from build123d import *

# Parameters (mm, degrees)
EXTRUDE_1_DEPTH     = 10
FILLET_1_R          = 5
CUT_EXTRUDE_1_DEPTH = 58.341084747
CUT_EXTRUDE_2_DEPTH = 59.557663888


with BuildPart() as part:
    # 草图1 → 凸台-拉伸1 (new body)
    with BuildSketch(Plane(origin=(0, 0, 0), x_dir=(0, 0, -1), z_dir=(1, 0, 0))):
        Polygon((0, 0), (52, 0), (52, 25), (49, 25), (49, 3), (3, 3), (3, 25), (0, 25), align=None)
    extrude(amount=EXTRUDE_1_DEPTH)

    # 圆角1
    fillet_1_edges = [part.edges().sort_by_distance(p)[0] for p in [
        (5, 3, -3),
        (5, 3, -49),
        (5, 0, -52),
        (5, 0, 0),
    ]]
    fillet(fillet_1_edges, radius=FILLET_1_R)

    # 草图2 → 切除-拉伸1 (cut, through all)
    with BuildSketch(Plane(origin=(0, 3, 0), x_dir=(1, 0, 0), z_dir=(0, 1, 0))):
        with BuildLine():
            Line((7.5, 33.5), (7.5, 18.5))
            ThreePointArc((7.5, 18.5), (5, 16), (2.5, 18.5))
            Line((2.5, 18.5), (2.5, 33.5))
            ThreePointArc((2.5, 33.5), (5, 36), (7.5, 33.5))
        make_face()
    extrude(amount=-CUT_EXTRUDE_1_DEPTH, mode=Mode.SUBTRACT)

    # 草图3 → 切除-拉伸2 (cut, through all)
    with BuildSketch(Plane.XY):
        with BuildLine():
            Line((7.5, 17.5), (7.5, 12.5))
            ThreePointArc((7.5, 12.5), (5, 10), (2.5, 12.5))
            Line((2.5, 12.5), (2.5, 17.5))
            ThreePointArc((2.5, 17.5), (5, 20), (7.5, 17.5))
        make_face()
    extrude(amount=-CUT_EXTRUDE_2_DEPTH, mode=Mode.SUBTRACT)


solid = part.part
Work out the finished part from the listing and answer in its coordinate system (mm). A direction names the side the tool comes from. Coordinates: 2 decimals unless noted, no trailing zeros. Loops run counter-clockwise (first coordinate to the right, second up) from the corner with the lowest first, then second, coordinate; pieces in that order, holes last. Notation, with made-up numbers: (21.25, -12) -> (80.25, -12) arc R10 cw to (80.25, 5) -> close; hole circle Ø8 at (-31, 86.5). An arc over 180 degrees is marked (long way). Answer as CSV lines item,"result".
1) For faces 4 (the face through (4.9, 20.2, -3)), 5 (the face through (2.5, 15, -50)), 6 (the face through (5, 2, -16)), determine the directions among +Z, -Z, +X, -X, +Y, -Y from which every point of the face is accessible in a straight line to the end or side of a thin tool.
A:
face 4,"+X, -X, +Y"
face 5,"+Z, -Z"
face 6,"+Y, -Y"
2) The part is cut by section A-A (x = 6.5). Give the vertices of the cut face in (y, z), and give its area (3 significant figures).
A:
outline,"(0, -47) arc R5 ccw to (5, -52) -> (10.5, -52) -> (10.5, -49) -> (8, -49) arc R5 cw to (3, -44) -> (3, -35.5) -> (0, -35.5) -> close; (0, -16.5) -> (3, -16.5) -> (3, -8) arc R5 cw to (8, -3) -> (10.5, -3) -> (10.5, 0) -> (5, 0) arc R5 ccw to (0, -5) -> close; (19.5, -52) -> (25, -52) -> (25, -49) -> (19.5, -49) -> close; (19.5, -3) -> (25, -3) -> (25, 0) -> (19.5, 0) -> close"
area,"177 mm²"
3) The part is cut by section D-D (y = 9). Give the vertices of the cut face in (x, z).
A:
outline,"(0, -52) -> (10, -52) -> (10, -49) -> (0, -49) -> close; (0, -3) -> (10, -3) -> (10, 0) -> (0, 0) -> close"
4) Flat-ended cylindrical pins translate along their axes: pin 1 (3 mm diameter, centred on x = 4, z = -34, fed in from +Y); pin 2 (1 mm diameter, centred on x = 5.5, y = 4, fed in from +Z). Find the tip coordinate at first contact, or state that the pin passes through.
A:
pin 1,"stops at y = 3"
pin 2,"stops at z = -0.03"
5) The part is cut by section C-C (z = -28). Give the vertices of the cut face in (x, y).
A:
outline,"(0, 0) -> (2.5, 0) -> (2.5, 3) -> (0, 3) -> close; (7.5, 0) -> (10, 0) -> (10, 3) -> (7.5, 3) -> close"
6) The part is cut by section B-B (y = 15.5). Give the vertices of the cut face in (x, z), and give its area (3 significant figures).
A:
outline,"(0, -52) -> (2.5, -52) -> (2.5, -49) -> (0, -49) -> close; (0, -3) -> (2.5, -3) -> (2.5, 0) -> (0, 0) -> close; (7.5, -52) -> (10, -52) -> (10, -49) -> (7.5, -49) -> close; (7.5, -3) -> (10, -3) -> (10, 0) -> (7.5, 0) -> close"
area,"30.0 mm²"
7) For a pull along Z with two mould halves and no side action, classify faces 1 (the face through (5, 10, -50)), 2 (the face through (7.5, 2, -26)), 3 (the face through (5, 1, -2)) as released by +Z, released by -Z, zero draft, split by the parting line, or undercut.
A:
face 1,"zero draft"
face 2,"undercut"
face 3,"released by +Z"
8) Straight lines are drawn through the part: probe 1 along Z at (x, y) = (2, 14.5); probe 2 along X at (y, z) = (13.5, -49.5); probe 3 along Y at (x, z) = (7.75, -36.5). For each, find the intervals that lie inside material, in ascending order.
A:
probe 1,"z = -52 to -49, -3 to 0"
probe 2,"x = 0 to 2.5, 7.5 to 10"
probe 3,"y = 0 to 3"
